Answer from the drawing. Dimensions are ordinates in mm from the lowest x, y and z of the part. Coordinates: 2 decimals unless noted, no trailing zeros. Write each loop counter-clockwise with the first axis right and the second up, starting at its lowest first coordinate (ties: lowest second). Pieces come first, ordered by that corner, then holes. Notation, with made-up numbers: (26, 45) - (70, 45) arc R21 cw to (70, 53) - close; hole circle Ø10 at (-22.5, 21.25). An arc over 180 degrees is marked (long way). Use CSV: the item, a comma, the result in double quotes. Start each with the question number.
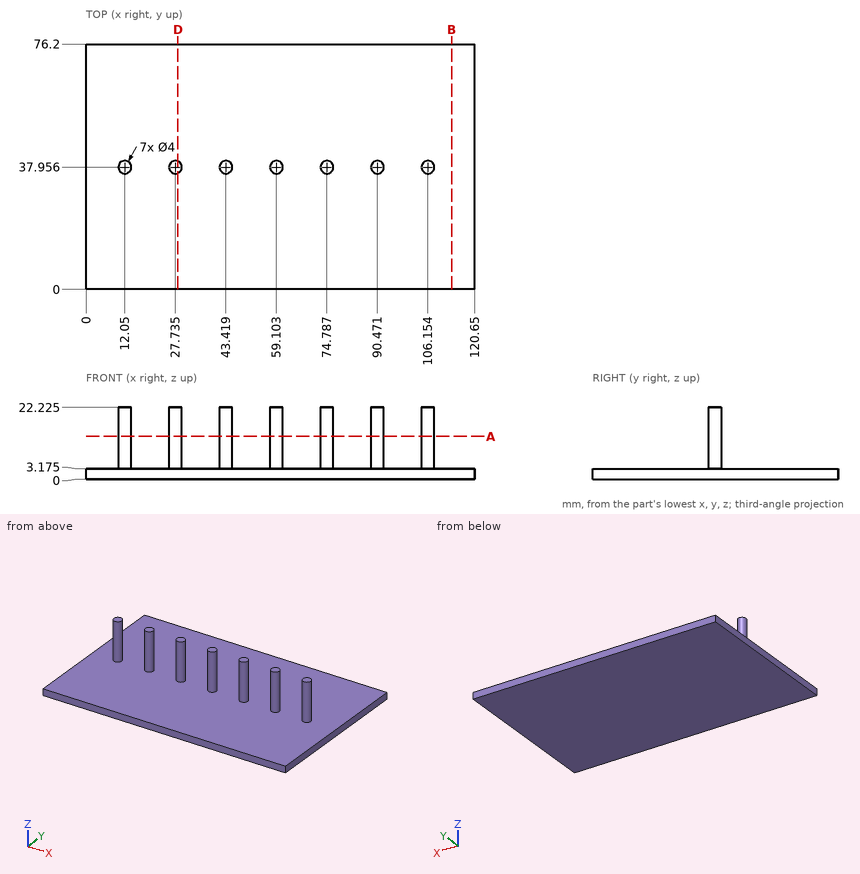
Item 1: A cutting plane is placed at B-B (x = 113.5). Determine the outline of the cut face in (y, z) (1 decimal).
Item 2: A cutting plane is placed at D-D (x = 28.5). Determine the outline of the cut face in (y, z) (1 decimal).
Item 3: Straight lines are drawn through the part: probe 1 along Z at (x, y) = (27, 7.5) (1 decimal); probe 2 along Y at (x, z) = (10.5, 16.5) (1 decimal); probe 3 along Y at (x, z) = (75.5, 5) (1 decimal). For each, find the intervals that lie inside material, in ascending order. Write a range as [from, to].
Item 4: Each of these flat-tipped pins is pushed along its axis until it touches: pin 1 (6 mm diameter, centred on x = 57, z = 16.5, fed in from -Y); pin 2 (2 mm diameter, centred on y = 37.5, z = 6.5, fed in from +X) (1 decimal); pin 3 (3 mm diameter, centred on x = 90, y = 21.5, fed in from +Z) (1 decimal). Where does it stop, or does it pass through?
Item 5: A cutting plane is placed at A-A (z = 13.25). Count the separate pieces of the cut face and the enclosed holes in it.
Calculated:
1,outline,"(0, 0) - (76.2, 0) - (76.2, 3.2) - (0, 3.2) - close"
2,outline,"(0, 0) - (76.2, 0) - (76.2, 3.2) - (39.8, 3.2) - (39.8, 22.2) - (36.1, 22.2) - (36.1, 3.2) - (0, 3.2) - close"
3,probe 1,"z = [0, 3.2]"
3,probe 2,"y = [36.7, 39.2]"
3,probe 3,"y = [36.1, 39.8]"
4,pin 1,"stops at y = 35.96"
4,pin 2,"stops at x = 108.2"
4,pin 3,"stops at z = 3.2"
5,separate pieces,"7"
5,enclosed holes,"0"
